Verification items for this drawing (mm, ordinates from the low corner). A direction names the side the tool comes from. Round coordinates to 2 decimals unless told otherwise and drop trailing zeros. Loops run counter-clockwise (first coordinate to the right, second up) from the corner with the lowest first, then second, coordinate; pieces in that order, holes last. Notation, with made-up numbers: M -40,48.5 L 12,48.5 A27 cw 12,76.5 Z; hole C 15,-9.5 d7. An arc over 180 degrees is marked long. Answer in a Markdown table with one row per item. Add a question column.
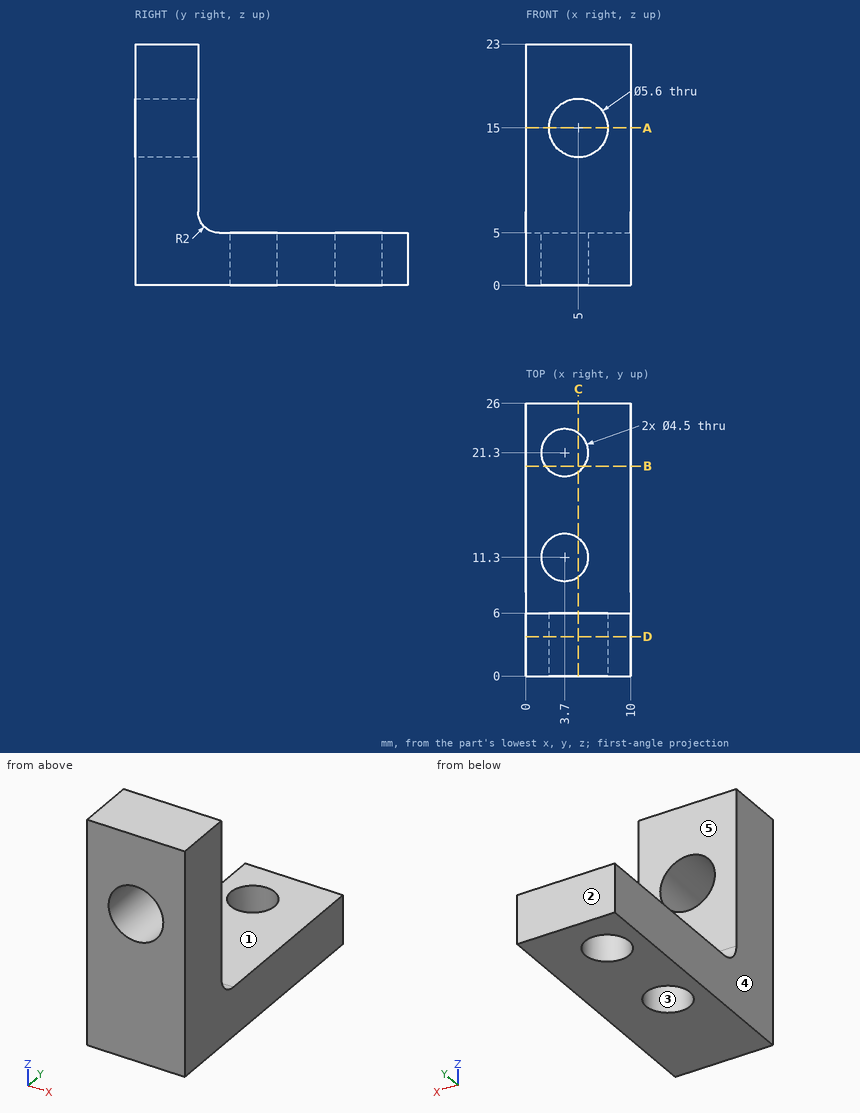
1) Set-up check for the marked faces 1 and 2: record each of +Z, -Z, +X, -X, +Y, -Y from which the full face is reachable in a straight line by a thin tool's end or side.
2) Thickness scan on L1, parallel to Y at x = 3.7, z = 3.35; L2, parallel to X at y = 2.65, z = 15; L3, parallel to Z at x = 6.25, y = 16.25. Record the ranges inside material, lowest first. Write a range as [from, to].
3) Cross-section at B-B, the plane y = 20. Record the boundary of the cut face in (x, z), plus the area to 3 significant figures.
4) Cross-section at C-C, the plane x = 5. Record the boundary of the cut face in (y, z).
5) Go/stop test with flat-tipped pins: pin 1 (1 mm diameter, centred on x = 2, y = 15.5, fed in from -Z); pin 2 (3.5 mm diameter, centred on x = 3.7, y = 21.3, fed in from +Z); pin 3 (5 mm diameter, centred on x = 4, y = 17, fed in from +Z); pin 4 (5 mm diameter, centred on x = 6, z = 14, fed in from +Y). Record where each tip stops, or that it passes through.
6) Cross-section at A-A, the plane z = 15. Record the boundary of the cut face in (x, y).
7) Draft check along X on the marked faces 3, 4 and 5. Enter one of: +X half, -X half, draft (parallel to the pull), parting line (faces both ways), or undercut.
8) Cross-section at D-D, the plane y = 3.75. Record the boundary of the cut face in (x, z).
Worked answers:
| question | item | result |
|---|---|---|
| 1 | face 1 | +Z, +X, -X, +Y |
| 1 | face 2 | +Z, -Z, +X, -X, +Y |
| 2 | L1 | y = [0, 9.05], [13.55, 19.05], [23.55, 26] |
| 2 | L2 | x = [0, 2.2], [7.8, 10] |
| 2 | L3 | z = [0, 5] |
| 3 | outline | M 0,0 L 1.86,0 L 1.86,5 L 0,5 Z; M 5.54,0 L 10,0 L 10,5 L 5.54,5 Z |
| 3 | area | 31.6 mm2 |
| 4 | outline | M 0,0 L 9.46,0 L 9.46,5 L 8,5 A2 cw 6,7 L 6,12.2 L 0,12.2 Z; M 0,17.8 L 6,17.8 L 6,23 L 0,23 Z; M 13.14,0 L 19.46,0 L 19.46,5 L 13.14,5 Z; M 23.14,0 L 26,0 L 26,5 L 23.14,5 Z |
| 5 | pin 1 | stops at z = 0 |
| 5 | pin 2 | passes through |
| 5 | pin 3 | stops at z = 5 |
| 5 | pin 4 | stops at y = 6 |
| 6 | outline | M 0,0 L 2.2,0 L 2.2,6 L 0,6 Z; M 7.8,0 L 10,0 L 10,6 L 7.8,6 Z |
| 7 | face 3 | undercut |
| 7 | face 4 | -X half |
| 7 | face 5 | draft |
| 8 | outline | M 0,0 L 10,0 L 10,23 L 0,23 Z; hole C 5,15 d5.6 |
